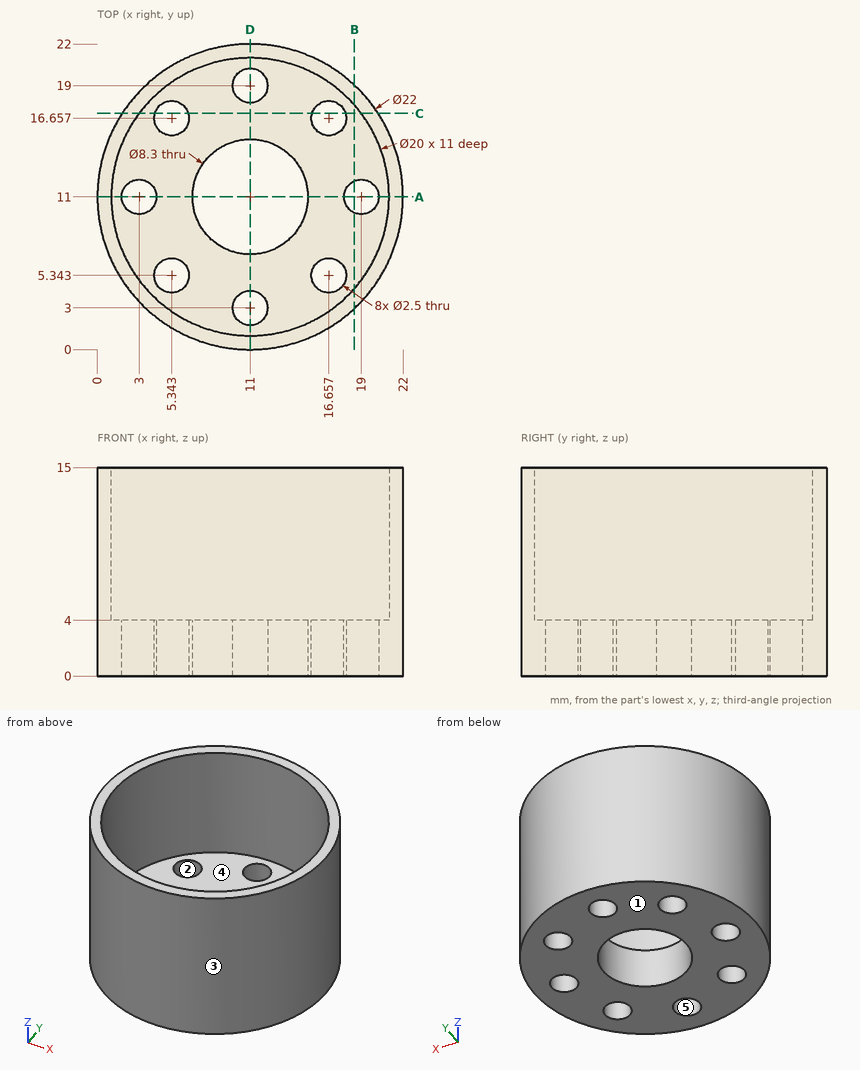
Verification items for this drawing (mm, ordinates from the low corner). A direction names the side the tool comes from. Coordinates: 2 decimals unless noted, no trailing zeros. Loops run counter-clockwise (first coordinate to the right, second up) from the corner with the lowest first, then second, coordinate; pieces in that order, holes last.
Item 1: Access from +Z, -Z, +X, -X, +Y, -Y to the whole of each face (thin tool, end or side, straight path). Record for the marked faces 4 and 5.
Item 2: Thickness scan on line 1 (Y direction, x = 11, z = 2.6); line 2 (X direction, y = 11.25, z = 6.5); line 3 (X direction, y = 4, z = 7.25) (1 decimal). Record the ranges inside material, lowest first.
Item 3: Sectioned sample at C-C, the plane y = 17. Record the boundary of the cut face in (x, z) (1 decimal).
Item 4: Go/stop test with flat-tipped pins: pin 1 Ø3 at (x, y) = (5.34, 16.66) entering from +Z; pin 2 Ø2 at (x, z) = (9.5, 9.5) entering from -Y; pin 3 Ø1 at (y, z) = (17.5, 11.5) entering from -X. Record where each tip stops, or that it passes through.
Item 5: Release check for a two-part mould opening along Y. For the marked faces 1, 2 and 3 record: released by +Y, released by -Y, zero draft, split by the parting line, or undercut.
Item 6: Sectioned sample at A-A, the plane y = 11. Record the boundary of the cut face in (x, z), then the cut area to 3 significant figures.
Item 7: Sectioned sample at B-B, the plane x = 18.5. Record the boundary of the cut face in (y, z).
Check result:
1. face 4: +Z
1. face 5: +Z, -Z
2. line 1: y = 0 to 1.75, 4.25 to 6.85, 15.15 to 17.75, 20.25 to 22
2. line 2: x = 0 to 1, 21 to 22
2. line 3: x = 2.5 to 3.9, 18.1 to 19.5
3. outline: (1.8, 0) - (4.1, 0) - (4.1, 4) - (3, 4) - (3, 15) - (1.8, 15) - close; (6.5, 0) - (15.5, 0) - (15.5, 4) - (6.5, 4) - close; (17.9, 0) - (20.2, 0) - (20.2, 15) - (19, 15) - (19, 4) - (17.9, 4) - close
4. pin 1: stops at z = 4
4. pin 2: stops at y = 0.01
4. pin 3: stops at x = 1.78
5. face 1: zero draft
5. face 2: undercut
5. face 3: split by the parting line
6. outline: (0, 0) - (1.75, 0) - (1.75, 4) - (1, 4) - (1, 15) - (0, 15) - close; (4.25, 0) - (6.85, 0) - (6.85, 4) - (4.25, 4) - close; (15.15, 0) - (17.75, 0) - (17.75, 4) - (15.15, 4) - close; (20.25, 0) - (22, 0) - (22, 15) - (21, 15) - (21, 4) - (20.25, 4) - close
6. area: 56.8 mm2
7. outline: (2.95, 0) - (9.85, 0) - (9.85, 4) - (4.39, 4) - (4.39, 15) - (2.95, 15) - close; (12.15, 0) - (19.05, 0) - (19.05, 15) - (17.61, 15) - (17.61, 4) - (12.15, 4) - close
